```python
from build123d import *

# Parameters (mm, degrees)
ESQUISSE1_W      = 25
ESQUISSE1_H      = 80
EXTRUSION1_DEPTH = 6
ESQUISSE2_R      = 8
ESQUISSE2_R_2    = 2.5
EXTRUSION2_DEPTH = 85.029756634
CHANFREIN1_SIZE  = 2


with BuildPart() as part:
    # Esquisse1 → Extrusion1 (new body)
    with BuildSketch(Plane(origin=(0, 0, 0), x_dir=(0, 0, -1), z_dir=(1, 0, 0))):
        with Locations((12.5, 40)):
            Rectangle(ESQUISSE1_W, ESQUISSE1_H)
    extrude(amount=EXTRUSION1_DEPTH)

    # Esquisse2 → Extrusion2 (cut, through all)
    with BuildSketch(Plane(origin=(6, 0, 0), x_dir=(0, 0, -1), z_dir=(1, 0, 0))):
        with Locations((15, 40)):
            Circle(ESQUISSE2_R)
        with Locations((5, 5)):
            Circle(ESQUISSE2_R_2)
        with Locations((18, 5)):
            Circle(ESQUISSE2_R_2)
        with Locations((5, 75)):
            Circle(ESQUISSE2_R_2)
        with Locations((18, 75)):
            Circle(ESQUISSE2_R_2)
    extrude(amount=-EXTRUSION2_DEPTH, mode=Mode.SUBTRACT)

    # Chanfrein1
    chanfrein1_edges = [part.edges().sort_by_distance(p)[0] for p in [
        (6, 5, -2.5),
        (6, 5, -15.5),
        (6, 75, -2.5),
        (6, 75, -15.5),
    ]]
    chamfer(chanfrein1_edges, length=CHANFREIN1_SIZE)


solid = part.part
```
For this review, take the finished solid that the model builds, in its own axes (mm). Round coordinates to 2 decimals unless told otherwise and drop trailing zeros. Write each loop counter-clockwise with the first axis right and the second up, starting at its lowest first coordinate (ties: lowest second). Pieces come first, ordered by that corner, then holes. Notation, with made-up numbers: (58.25, 53) -> (103.25, 53) arc R19 cw to (103.25, 82) -> close; hole circle Ø2 at (-38.75, 13.25). An arc over 180 degrees is marked (long way). One line per question, with ' | ' between items. Start each with the question number.
1) Mouldability with a two-part tool opening along Z and no side actions: class faces 1 (the flat face through (0, 40.6, -6.8)), 2 (the cylindrical face through (2.028, 5.751, -7.385)), 3 (the flat face through (3, 39, 0)), 4 (the flat face through (3, 39, -25)) as +Z half, -Z half, draft (parallel to the pull), parting line (faces both ways), or undercut.
2) Add section C-C (z = -5). Write out the cut boundary in (x, y), and give its area (3 significant figures).
3) Wall thickness on line 1 along Y through (x, z) = (3, -5); line 2 along Z through (x, y) = (4.05, 75); line 3 along Y through (x, z) = (3.05, -18): over which ranges is each line inside the solid? List them lowest first.
4) For pin 1 Ø6.5 at (y, z) = (75, -5) entering from +X, flat-tipped, find the tip position at first contact; note if it passes through.
5) Add section B-B (y = 75). Write out the cut boundary in (x, z), and give its area (3 significant figures).
6) Add section A-A (x = 2.45). Write out the cut boundary in (y, z), and give its area (3 significant figures).
7) Add section D-D (y = 40). Write out the cut boundary in (x, z), and give its area (3 significant figures).
Reported:
1) face 1: draft | face 2: undercut | face 3: +Z half | face 4: -Z half
2) outline: (0, 0) -> (6, 0) -> (6, 0.5) -> (4, 2.5) -> (0, 2.5) -> close; (0, 7.5) -> (4, 7.5) -> (6, 9.5) -> (6, 70.5) -> (4, 72.5) -> (0, 72.5) -> close; (0, 77.5) -> (4, 77.5) -> (6, 79.5) -> (6, 80) -> (0, 80) -> close | area: 412 mm²
3) line 1: y = 0 to 2.5, 7.5 to 72.5, 77.5 to 80 | line 2: z = -25 to -20.55, -15.45 to -7.55, -2.45 to 0 | line 3: y = 0 to 2.5, 7.5 to 32.58, 47.42 to 72.5, 77.5 to 80
4) pin 1: stops at x = 4.75
5) outline: (0, -25) -> (6, -25) -> (6, -22.5) -> (4, -20.5) -> (0, -20.5) -> close; (0, -15.5) -> (4, -15.5) -> (6, -13.5) -> (6, -9.5) -> (4, -7.5) -> (0, -7.5) -> close; (0, -2.5) -> (4, -2.5) -> (6, -0.5) -> (6, 0) -> (0, 0) -> close | area: 82.0 mm²
6) outline: (0, -25) -> (80, -25) -> (80, 0) -> (0, 0) -> close; hole circle Ø5 at (5, -18); hole circle Ø5 at (5, -5); hole circle Ø16 at (40, -15); hole circle Ø5 at (75, -18); hole circle Ø5 at (75, -5) | area: 1,720 mm²
7) outline: (0, -25) -> (6, -25) -> (6, -23) -> (0, -23) -> close; (0, -7) -> (6, -7) -> (6, 0) -> (0, 0) -> close | area: 54.0 mm²
